from build123d import *

# Parameters (mm, degrees)
SKETCH1_R           = 20
BOSS_EXTRUDE1_DEPTH = 71
SKETCH2_R           = 7.5
BOSS_EXTRUDE2_DEPTH = 1.4
SKETCH3_R           = 4.5
BOSS_EXTRUDE3_DEPTH = 2.15
SKETCH4_R           = 3
BOSS_EXTRUDE4_DEPTH = 16.75
SKETCH5_R           = 1.5
CUT_EXTRUDE1_DEPTH  = 5
CIRPATTERN1_COUNT   = 6
BOSS_EXTRUDE5_DEPTH = 18.73


with BuildPart() as part:
    # Sketch1 → Boss-Extrude1 (new body)
    with BuildSketch(Plane(origin=(0, 0, 0), x_dir=(1, 0, 0), z_dir=(0, 1, 0))):
        Circle(SKETCH1_R)
    extrude(amount=BOSS_EXTRUDE1_DEPTH)

    # Sketch2 → Boss-Extrude2 (add)
    with BuildSketch(Plane(origin=(0, 71, 0), x_dir=(1, 0, 0), z_dir=(0, 1, 0))):
        Circle(SKETCH2_R)
    extrude(amount=BOSS_EXTRUDE2_DEPTH)

    # Sketch3 → Boss-Extrude3 (add)
    with BuildSketch(Plane(origin=(0, 72.4, 0), x_dir=(1, 0, 0), z_dir=(0, 1, 0))):
        Circle(SKETCH3_R)
    extrude(amount=BOSS_EXTRUDE3_DEPTH)

    # Sketch4 → Boss-Extrude4 (add)
    with BuildSketch(Plane(origin=(0, 74.55, 0), x_dir=(1, 0, 0), z_dir=(0, 1, 0))):
        Circle(SKETCH4_R)
    extrude(amount=BOSS_EXTRUDE4_DEPTH)

    # Sketch5 → Cut-Extrude1 (cut)
    with BuildSketch(Plane(origin=(0, 71, 0), x_dir=(1, 0, 0), z_dir=(0, 1, 0))):
        with Locations((-11, 0)):
            Circle(SKETCH5_R)
    cut_extrude1 = extrude(amount=-CUT_EXTRUDE1_DEPTH, mode=Mode.SUBTRACT)

    # CirPattern1: Cut-Extrude1 ×6 about axis
    cirpattern1_axis = Axis((0, 0, 0), (0, 1, 0))
    for i in range(1, CIRPATTERN1_COUNT):
        add(cut_extrude1.rotate(cirpattern1_axis, i * 360 / CIRPATTERN1_COUNT), mode=Mode.SUBTRACT)

    # Sketch6 → Boss-Extrude5 (add)
    with BuildSketch(Plane(origin=(0, 0, 0), x_dir=(-1, 0, 0), z_dir=(0, -1, 0))):
        with BuildLine():
            Line((15, 0), (15, 25))
            Line((15, 25), (-15, 25))
            Line((-15, 25), (-15, 0))
            ThreePointArc((-15, 0), (0, -15), (15, 0))
        make_face()
    extrude(amount=BOSS_EXTRUDE5_DEPTH)


solid = part.part
Work out the finished part from the listing and answer in its coordinate system (mm). A direction names the side the tool comes from. Coordinates: 2 decimals unless noted, no trailing zeros. Order: outer loops, then holes, each group sorted by start corner. A loop starts at its lowest first (then second) coordinate and runs counter-clockwise, first axis right, second up. Notation, with made-up numbers: (12.5, -4) - (52.5, -4) arc R28 cw to (52.5, 31) - close; hole circle Ø4 at (6.25, -11.5). An arc over 180 degrees is marked (long way). Put each result on its own line as item: value. Start each with the question number.
1) Find the intervals of material crossed by line 1 (Z direction, x = 5.5, y = 69.95); line 2 (Y direction, x = 6, z = 4); line 3 (Z direction, x = 5, y = 68), in increasing order. Write a range as from..to.
2) Find section B-B (y = 54.5). Give the vertices of the cut face in (x, z).
3) For faces 4 (the flat face through (0, 71, 9)), 5 (the cylindrical face through (0, -9, 15)), 6 (the flat face through (0, 91.3, 0)), determine the directions among +Z, -Z, +X, -X, +Y, -Y from which every point of the face is accessible in a straight line to the end or side of a thin tool.
4) Find section C-C (x = -11). Give the vertices of the cut face in (y, z), plus the area to 3 significant figures.
5) Flat-ended cylindrical pins translate along their axes: pin 1 (2.5 mm diameter, centred on x = -6, z = 9.5, fed in from +Y); pin 2 (1 mm diameter, centred on x = 7, y = 57, fed in from -Z); pin 3 (2 mm diameter, centred on y = 45.5, z = 2, fed in from +X) (3 decimals). Find the tip coordinate at first contact, or state that the pin passes through.
6) For a pull along Z with two mould halves and no side action, classify faces 1 (the flat face through (6, 66, -10)), 2 (the flat face through (0, -18.73, -5)), 3 (the cylindrical face through (-0.59, 73.46, -4.46)) as released by +Z, released by -Z, zero draft, split by the parting line, or undercut.
7) Find section A-A (x = 0). Give the vertices of the cut face in (y, z).
8) Find section D-D (x = 17). Give the vertices of the cut face in (y, z), plus the area to 3 significant figures.
Results list:
1. line 1: z = -19.23..-11.03, -8.03..8.03, 11.03..19.23
1. line 2: y = -18.73..72.4
1. line 3: z = -19.36..-10.94, -8.11..8.11, 10.94..19.36
2. outline: circle Ø40 at (0, 0)
3. face 4: +Y
3. face 5: +Z, -Y
3. face 6: +Z, -Z, +X, -X, +Y
4. outline: (-18.73, -25) - (0, -25) - (0, -16.7) - (71, -16.7) - (71, -1.5) - (66, -1.5) - (66, 1.5) - (71, 1.5) - (71, 16.7) - (0, 16.7) - (0, 10.2) - (-18.73, 10.2) - close
4. area: 3,020 mm^2
5. pin 1: stops at y = 71
5. pin 2: stops at z = -18.91
5. pin 3: stops at x = 19.975
6. face 1: undercut
6. face 2: zero draft
6. face 3: split by the parting line
7. outline: (-18.73, -25) - (0, -25) - (0, -20) - (71, -20) - (71, -7.5) - (72.4, -7.5) - (72.4, -4.5) - (74.55, -4.5) - (74.55, -3) - (91.3, -3) - (91.3, 3) - (74.55, 3) - (74.55, 4.5) - (72.4, 4.5) - (72.4, 7.5) - (71, 7.5) - (71, 20) - (0, 20) - (0, 15) - (-18.73, 15) - close
8. outline: (0, -10.54) - (71, -10.54) - (71, 10.54) - (0, 10.54) - close
8. area: 1,500 mm^2
